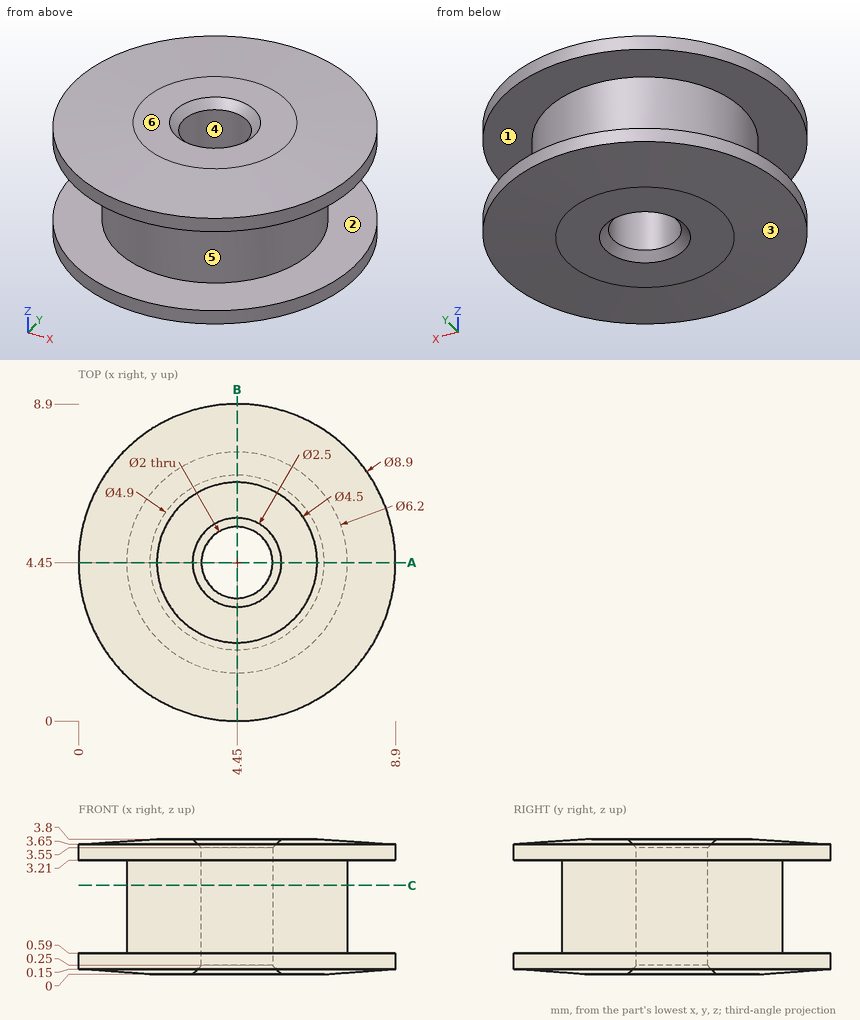
Design review of the part shown in the three views and the two pictorial views. Dimensions are in mm from the part's minimum x, y and z. A direction names the side the tool comes from. Coordinates: 2 decimals unless noted, no trailing zeros. Order: outer loops, then holes, each group sorted by start corner. A loop starts at its lowest first (then second) coordinate and runs counter-clockwise, first axis right, second up. Notation, with made-up numbers: (-2, 61) - (3, 61) arc R17 cw to (3, 73) - close; hole circle Ø4 at (33, 37.25). An arc over 180 degrees is marked (long way). Answer as CSV lines item,"result". Start each with the question number.
1) Machinability: for the marked faces 5 and 6, which of the approach directions +Z, -Z, +X, -X, +Y, -Y give a long, thin tool a straight path to every point of the face, cutting with its end or side? Answer none if there is none.
2) Draft analysis for pull direction Z (two halves, no side actions). For the marked faces 1, 2, 3 and 4, state which applies: +Z half, -Z half, draft (parallel to the pull), parting line (faces both ways), or undercut.
3) Add section C-C (z = 2.5). State the section outline as (x, y) points.
4) Insertion check: P1, Ø1, axis at x = 8, y = 6.5, coming from the +Z side; P2, Ø1, axis at y = 6.5, z = 2.5, coming from the -X side; P3, Ø2, axis at y = 5.5, z = 1.5, coming from the +X side; P4, Ø5, axis at x = 6, y = 1, coming from the +Z side. Each pin has a flat end and moves straight along its axis. Give the tip position at first contact, or say it passes through.
5) To check wall thickness, follow line 1 along Y through (x, z) = (4.45, 2.35); line 2 along X through (y, z) = (5.25, 2.05) (3 decimals); line 3 along Z through (x, y) = (6.25, 1.5). State the ranges of each line that lie inside material, in increasing order. Write a range as [from, to].
6) Add section A-A (y = 4.45). State the section outline as (x, z) points, then the cut area to 3 significant figures.
Result:
1,face 5,"none"
1,face 6,"+Z, +X, -X, +Y, -Y"
2,face 1,"undercut"
2,face 2,"undercut"
2,face 3,"-Z half"
2,face 4,"draft"
3,outline,"circle Ø6.2 at (4.45, 4.45); hole circle Ø2 at (4.45, 4.45)"
4,P1,"z = 3.71"
4,P2,"x = 1.77"
4,P3,"x = 8.85"
4,P4,"z = 3.8"
5,line 1,"[1.35, 3.45], [5.45, 7.55]"
5,line 2,"[1.455, 3.85], [5.05, 7.445]"
5,line 3,"[0.08, 0.59], [3.21, 3.72]"
6,outline,"(0, 0.15) - (2, 0) - (3.2, 0) - (3.45, 0.25) - (3.45, 3.55) - (3.2, 3.8) - (2.2, 3.8) - (0, 3.65) - (0, 3.21) - (1.35, 3.21) - (1.35, 0.59) - (0, 0.59) - close; (5.45, 0.25) - (5.7, 0) - (6.9, 0) - (8.9, 0.15) - (8.9, 0.59) - (7.55, 0.59) - (7.55, 3.21) - (8.9, 3.21) - (8.9, 3.65) - (6.7, 3.8) - (5.7, 3.8) - (5.45, 3.55) - close"
6,area,"18.4 mm^2"
